Input: part model. Units: mm. Frame: model coordinates. A direction names the side the tool comes from. Coordinates: 2 decimals unless noted, no trailing zeros. Write each loop counter-clockwise with the first axis right and the second up, starting at its lowest first coordinate (ties: lowest second). Pieces come first, ordered by that corner, then holes. Notation, with made-up numbers: M 73.25,-27.5 L 128.25,-27.5 A22 cw 128.25,5.5 Z; hole C 50,61.25 d4. An arc over 180 degrees is marked long. Answer as a JSON object with one key per item and string values. Group by question number.
from build123d import *

# Parameters (mm, degrees)
F1_DEPTH = 5
F3_DEPTH = 25
F5_R     = 10
F6_DEPTH = 40.2
F7_R     = 0.5


with BuildPart() as f1:
    # F0 (on Top) → F1 (new body)
    with BuildSketch(Plane.XY):
        with BuildLine():
            ThreePointArc((-4.8529455066, -11.3703208044), (-9.7372457817, 13.1811290021), (-12.094983449, 38.1024281231))
            ThreePointArc((-12.094983449, 38.1024281231), (-25.1726018808, 39.2244660439), (-38.1818190217, 37.4799482524))
            ThreePointArc((-38.1818190217, 37.4799482524), (-57.5543992317, 16.3508865245), (-64.8529455066, -11.3703208044))
            ThreePointArc((-64.8529455066, -11.3703208044), (-34.8529455066, -14.6827008575), (-4.8529455066, -11.3703208044))
        make_face()
    extrude(amount=F1_DEPTH)

    # F2 (on face) → F3 (cut)
    with BuildSketch(Plane.XY.offset(5)):
        with BuildLine():
            Line((-10.445380618, 18.4103436768), (-14.0728279948, 18.4103436768))
            Line((-14.0728279948, 18.4103436768), (-14.0728279948, 16.4103436768))
            Line((-14.0728279948, 16.4103436768), (-10.1880609939, 16.4103436768))
            ThreePointArc((-10.1880609939, 16.4103436768), (-10.3187750863, 17.4100793735), (-10.445380618, 18.4103436768))
        make_face()
        with BuildLine():
            ThreePointArc((-9.2078046903, 9.7353123128), (-9.3665647814, 10.7349891474), (-9.521200175, 11.7353123128))
            Line((-9.521200175, 11.7353123128), (-13.6872706935, 11.7353123128))
            Line((-13.6872706935, 11.7353123128), (-13.6872706935, 9.7353123128))
            Line((-13.6872706935, 9.7353123128), (-9.2078046903, 9.7353123128))
        make_face()
        with BuildLine():
            Line((-25.4467576742, -11.0847614706), (-25.4467576742, -14.3606151844))
            ThreePointArc((-25.4467576742, -14.3606151844), (-24.4464809139, -14.2883663577), (-23.4467576742, -14.2088243302))
            Line((-23.4467576742, -14.2088243302), (-23.4467576742, -11.0847614706))
            Line((-23.4467576742, -11.0847614706), (-25.4467576742, -11.0847614706))
        make_face()
        with BuildLine():
            ThreePointArc((-20.0489610434, -13.8834992945), (-19.0485375374, -13.7714603365), (-18.0489610434, -13.6521005786))
            Line((-18.0489610434, -13.6521005786), (-18.0489610434, -9.9280904979))
            Line((-18.0489610434, -9.9280904979), (-20.0489610434, -9.9280904979))
            Line((-20.0489610434, -9.9280904979), (-20.0489610434, -13.8834992945))
        make_face()
    extrude(amount=-F3_DEPTH, mode=Mode.SUBTRACT)

    # F5 (on face) → F6 (cut)
    with BuildSketch(Plane.XY.offset(5)):
        with Locations((-46.07405141, 2.2169523872)):
            Circle(F5_R)
        with Locations((-31.8084470928, 23.4225839376)):
            Circle(F5_R)
    extrude(amount=-F6_DEPTH, mode=Mode.SUBTRACT)

    # F7
    f7_edges = [f1.edges().sort_by_distance(p)[0] for p in [
        (-4.852946, -11.370321, 2.5),
        (-64.852946, -11.370321, 2.5),
        (-12.094983, 38.102428, 2.5),
        (-38.181819, 37.479948, 2.5),
    ]]
    fillet(f7_edges, radius=F7_R)


solid = f1.part
Q1. Pin query (flat end, axial travel): pin 1 Ø1.6 at (x, z) = (-24.5, 3) entering from -Y; pin 2 Ø1 at (x, z) = (-19, 2) entering from -Y; pin 3 Ø1.6 at (y, z) = (17.5, 1.5) entering from +X. Return the tip coordinate at first contact, or that it passes through.
Q2. Access query for faces 4 (the flat face through (-12, 18.41, 3)), 5 (the flat face through (-25.447, -13, 3)), 6 (the cylindrical face through (-11.77, -12.73, 2.46)). Directions: +Z, -Z, +X, -X, +Y, -Y. A direction counts if a zero-diameter tool reaches every point of the face in a straight line with its end or side. Return the directions, or none.
Q3. Section B-B, the plane y = -1.5. Return the cut outline in (x, z), and give its area (3 significant figures).
Q4. Line query: line 1 (Y direction, x = -13, z = 0.7); line 2 (Y direction, x = -40, z = 1.25); line 3 (X direction, y = 6, z = 1.35). Output: solid intervals per line, ascending. Write a range as from..to.
Q5. Draft query along Y for faces 1 (the cylindrical face through (-21.77, -14.06, 2.46)), 2 (the cylindrical face through (-7.284, -0.758, 2.465)), 3 (the flat face through (-12, 11.735, 3)). Return one class per face: released by +Y, released by -Y, zero draft, split by the parting line, or undercut.
Q6. Section C-C, the plane z = 2.65. State how many separate pieces and enclosed holes the cut face has, and give its area (3 significant figures).
Q7. Section D-D, the plane x = -8.5. Return the cut outline in (y, z), and give its area (3 significant figures).
Q8. Section A-A, the plane x = -43. Return the cut outline in (y, z).
Filled in:
{
 "1": {"pin 1": "y = -11.08", "pin 2": "y = -9.93", "pin 3": "x = -14.07"},
 "2": {"face 4": "+Z, -Z, +X", "face 5": "+Z, -Z, -Y", "face 6": "+Z, -Z, +X, -Y"},
 "3": {"outline": "M -63.88,0 L -55.36,0 L -55.36,5 L -63.88,5 Z; M -36.79,0 L -7.13,0 L -7.13,5 L -36.79,5 Z", "area": "191 mm^2"},
 "4": {"line 1": "-12.94..9.74, 11.74..16.41, 18.41..38.27", "line 2": "-14.59..-5.73, 10.16..17.69, 29.16..36.22", "line 3": "-62..-55.33, -36.82..-8.58"},
 "5": {"face 1": "released by -Y", "face 2": "released by +Y", "face 3": "undercut"},
 "6": {"separate pieces": "1", "enclosed holes": "2", "area": "1,830 mm^2"},
 "7": {"outline": "M -12.13,0 L 5.57,0 L 5.57,5 L -12.13,5 Z", "area": "88.5 mm^2"},
 "8": {"outline": "M -14.44,0 L -7.3,0 L -7.3,5 L -14.44,5 Z; M 11.73,0 L 33.92,0 L 33.92,5 L 11.73,5 Z"}
}
